```python
from build123d import *

# Parameters (mm, degrees)
F1_DEPTH = 19.05
F2_W     = 3.81
F2_H     = 3.175
F3_DEPTH = 5.588
F5_DEPTH = 7.113
F6_R     = 0.508
F7_DEPTH = 19.051


with BuildPart() as f1:
    # F0 (on Right) → F1 (new body)
    with BuildSketch(Plane.YZ):
        Polygon((-1.016, 1.27), (-1.016, 0), (1.016, 0), (1.016, 1.27), (2.5908, 1.27), (2.5908, 0), (3.4798, 0), (3.4798, 1.524), (8.5598, 1.524), (8.5598, 7.112), (-8.5598, 7.112), (-8.5598, 1.524), (-3.4798, 1.524), (-3.4798, 0), (-2.5908, 0), (-2.5908, 1.27), align=None)
    extrude(amount=-F1_DEPTH)

    # F2 (on face) → F3 (join, through all)
    with BuildSketch(Plane.XY.offset(7.112)):
        with Locations((-17.145, 10.1473)):
            Rectangle(F2_W, F2_H)
        with Locations((-17.145, -10.1473)):
            Rectangle(F2_W, F2_H)
    extrude(amount=-F3_DEPTH)

    # F4 (on face) → F5 (cut, through all)
    with BuildSketch(Plane.XY.offset(7.112)):
        with BuildLine():
            Line((0, -8.5598), (0, 8.5598))
            ThreePointArc((0, 8.5598), (-1.154422, 4.79553), (-1.645787, 0.889))
            Line((-1.645787, 0.889), (-1.137787, 0))
            Line((-1.137787, 0), (-1.645787, -0.889))
            ThreePointArc((-1.645787, -0.889), (-1.154422, -4.79553), (0, -8.5598))
        make_face()
    extrude(amount=-F5_DEPTH, mode=Mode.SUBTRACT)

    # F6 (on Right) → F7 (cut, through all)
    with BuildSketch(Plane.YZ):
        with Locations((0, 4.318)):
            Circle(F6_R)
    extrude(amount=-F7_DEPTH, mode=Mode.SUBTRACT)


solid = f1.part
```
Design review of the part built by this model. Coordinates are the model's own, in mm. A direction names the side the tool comes from. Give positions to 0.01 mm unless a question says otherwise; leave off trailing zeros. Order: outer loops, then holes, each group sorted by start corner. A loop starts at its lowest first (then second) coordinate and runs counter-clockwise, first axis right, second up. Notation, with made-up numbers: (87, 50) - (104, 50) arc R26 ccw to (104, 72) - close; hole circle Ø11 at (32.25, 68). An arc over 180 degrees is marked (long way). Use a Markdown table: item, result. Add a question column.
(1) Mouldability with a two-part tool opening along Z and no side actions: class faces 1 (the face through (-10, 0, 7.112)), 2 (the face through (-12, -7, 1.524)), 3 (the face through (-8, 8.56, 4)), 4 (the face through (-9.97, -0.07, 4.82)) as +Z half, -Z half, draft (parallel to the pull), parting line (faces both ways), or undercut.
(2) Add section B-B on x = -7.25. Give the boundary of the cut face in (y, z), then the cut area to 3 significant figures.
(3) Clearance check with flat-ended pins moving along their axes: P1, Ø1.5, axis at y = -3, z = 5.5, coming from the +X side; P2, Ø4, axis at x = -13, y = -8, coming from the -Z side; P3, Ø0.8, axis at x = -7, y = 1.5, coming from the -Z side. State where each tip first meets the part, or that it passes through.
(4) Wall thickness on probe 1 along Y at (x, z) = (-9.25, 0.75); probe 2 along Z at (x, y) = (-15.5, 0); probe 3 along Z at (x, y) = (-11.25, 1.5): over which ranges is each line inside the solid? List them lowest first. Write a range as [from, to].
(5) Machinability: for faces 5 (the face through (-1.39, -0.44, 3.61)), 6 (the face through (-10, 3, 0)), 7 (the face through (-12, 7, 1.524)), 8 (the face through (-10, 2.591, 1)), 9 (the face through (-19.05, -0.2, 3.6)), which of the approach directions +Z, -Z, +X, -X, +Y, -Y give a long, thin tool a straight path to every point of the face, cutting with its end or side? Answer none if there is none.
(6) Add section C-C on y = 10.25. Give the boundary of the cut face in (x, z), then the cut area to 3 significant figures.
(7) Add section A-A on z = 5.75. Give the boundary of the cut face in (x, y), then the cut area to 3 significant figures.
(8) Add section D-D on x = -16. Give the boundary of the cut face in (y, z), then the cut area to 3 significant figures.
Report:
| question | item | result |
|---|---|---|
| 1 | face 1 | +Z half |
| 1 | face 2 | -Z half |
| 1 | face 3 | draft |
| 1 | face 4 | undercut |
| 2 | outline | (-8.56, 1.52) - (-3.48, 1.52) - (-3.48, 0) - (-2.59, 0) - (-2.59, 1.27) - (-1.02, 1.27) - (-1.02, 0) - (1.02, 0) - (1.02, 1.27) - (2.59, 1.27) - (2.59, 0) - (3.48, 0) - (3.48, 1.52) - (8.56, 1.52) - (8.56, 7.11) - (-8.56, 7.11) - close; hole circle Ø1.02 at (0, 4.32) |
| 2 | area | 101 mm² |
| 3 | P1 | stops at x = -1.35 |
| 3 | P2 | stops at z = 1.52 |
| 3 | P3 | stops at z = 1.27 |
| 4 | probe 1 | y = [-3.48, -2.59], [-1.02, 1.02], [2.59, 3.48] |
| 4 | probe 2 | z = [0, 3.81], [4.83, 7.11] |
| 4 | probe 3 | z = [1.27, 7.11] |
| 5 | face 5 | +Z, -Z, +X |
| 5 | face 6 | -Z, +X, -X, +Y, -Y |
| 5 | face 7 | -Z, +X, -X, +Y |
| 5 | face 8 | -Z, +X, -X |
| 5 | face 9 | +Z, -Z, -X, +Y, -Y |
| 6 | outline | (-19.05, 1.52) - (-15.24, 1.52) - (-15.24, 7.11) - (-19.05, 7.11) - close |
| 6 | area | 21.3 mm² |
| 7 | outline | (-19.05, -11.73) - (-15.24, -11.73) - (-15.24, -8.56) - (0, -8.56) arc R22.86 cw to (-1.65, -0.89) - (-1.14, 0) - (-1.65, 0.89) arc R22.86 cw to (0, 8.56) - (-15.24, 8.56) - (-15.24, 11.73) - (-19.05, 11.73) - close |
| 7 | area | 332 mm² |
| 8 | outline | (-11.73, 1.52) - (-3.48, 1.52) - (-3.48, 0) - (-2.59, 0) - (-2.59, 1.27) - (-1.02, 1.27) - (-1.02, 0) - (1.02, 0) - (1.02, 1.27) - (2.59, 1.27) - (2.59, 0) - (3.48, 0) - (3.48, 1.52) - (11.73, 1.52) - (11.73, 7.11) - (-11.73, 7.11) - close; hole circle Ø1.02 at (0, 4.32) |
| 8 | area | 137 mm² |
